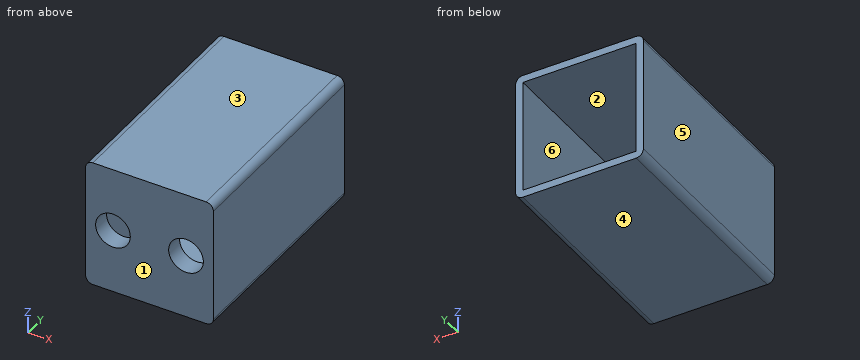
from build123d import *

# Parameters (mm, degrees)
SKETCH1_R           = 4.75
BOSS_EXTRUDE1_DEPTH = 60
SKETCH2_W           = 31
SKETCH2_H           = 31
CUT_EXTRUDE1_DEPTH  = 55


with BuildPart() as part:
    # Sketch1 → Boss-Extrude1 (new body)
    with BuildSketch(Plane(origin=(0, 0, 0), x_dir=(1, 0, 0), z_dir=(0, 1, 0))):
        with BuildLine():
            Line((2, 0), (33, 0))
            ThreePointArc((33, 0), (34.414213562, 0.585786438), (35, 2))
            Line((35, 2), (35, 33))
            ThreePointArc((35, 33), (34.414213562, 34.414213562), (33, 35))
            Line((33, 35), (2, 35))
            ThreePointArc((2, 35), (0.585786438, 34.414213562), (0, 33))
            Line((0, 33), (0, 2))
            ThreePointArc((0, 2), (0.585786438, 0.585786438), (2, 0))
        make_face()
        with Locations((7.5, 17.5)):
            Circle(SKETCH1_R, mode=Mode.SUBTRACT)
        with Locations((27.5, 17.5)):
            Circle(SKETCH1_R, mode=Mode.SUBTRACT)
    extrude(amount=BOSS_EXTRUDE1_DEPTH)

    # Sketch2 → Cut-Extrude1 (cut)
    with BuildSketch(Plane(origin=(0, 60, 0), x_dir=(1, 0, 0), z_dir=(0, 1, 0))):
        with Locations((17.5, 17.5)):
            Rectangle(SKETCH2_W, SKETCH2_H)
    extrude(amount=-CUT_EXTRUDE1_DEPTH, mode=Mode.SUBTRACT)


solid = part.part
CAD build for the part. Positions are in the model's coordinates, mm. Face numbers are marked on the shaded views. A direction names the side the tool comes from. Round coordinates to 2 decimals unless told otherwise and drop trailing zeros. Loops run counter-clockwise (first coordinate to the right, second up) from the corner with the lowest first, then second, coordinate; pieces in that order, holes last.
(1) Drop a flat-ended pin along its axis: pin 1 (1.5 mm diameter, centred on x = 29.5, z = -31.5, fed in from +Y). Give the stop position or say it passes through.
(2) Cut at D-D (z = -6.5). Give the cut face in (x, y), plus the area to 3 significant figures.
(3) Wall check: line 1 along X through (y, z) = (1.75, -17.5); line 2 along X through (y, z) = (9.5, -21.5); line 3 along Z through (x, y) = (7, 23). Give the ranges that are in metal, low to high.
(4) Which spindle directions (+Z, -Z, +X, -X, +Y, -Y) get a long thin tool onto all of the face, cutting with end or side? Do the marked faces 1 and 2. Say none if no direction does.
(5) Cut at A-A (x = 27.5). Give the cut face in (y, z), plus the area to 4 significant figures.
(6) Two-plate mould, pull along Z, no slides. Class the marked faces 3, 4, 5 and 6: +Z half, -Z half, draft (parallel to the pull), parting line (faces both ways), or undercut.
(7) Cut at C-C (y = 34.5). Give the cut face in (x, z), plus the area to 3 significant figures.
(8) Cut at B-B (z = -17.5). Give the cut face in (x, y).
Findings below:
1. pin 1: stops at y = 5
2. outline: (0, 0) - (35, 0) - (35, 60) - (33, 60) - (33, 5) - (2, 5) - (2, 60) - (0, 60) - close
2. area: 395 mm2
3. line 1: x = 0 to 2.75, 12.25 to 22.75, 32.25 to 35
3. line 2: x = 0 to 2, 33 to 35
3. line 3: z = -35 to -33, -2 to 0
4. face 1: +Z, -Z, +X, -X, -Y
4. face 2: +Y
5. outline: (0, -35) - (60, -35) - (60, -33) - (5, -33) - (5, -22.25) - (0, -22.25) - close; (0, -12.75) - (5, -12.75) - (5, -2) - (60, -2) - (60, 0) - (0, 0) - close
5. area: 347.5 mm2
6. face 3: +Z half
6. face 4: -Z half
6. face 5: draft
6. face 6: undercut
7. outline: (0, -33) arc R2 ccw to (2, -35) - (33, -35) arc R2 ccw to (35, -33) - (35, -2) arc R2 ccw to (33, 0) - (2, 0) arc R2 ccw to (0, -2) - close; hole (2, -33) - (33, -33) - (33, -2) - (2, -2) - close
7. area: 261 mm2
8. outline: (0, 0) - (2.75, 0) - (2.75, 5) - (2, 5) - (2, 60) - (0, 60) - close; (12.25, 0) - (22.75, 0) - (22.75, 5) - (12.25, 5) - close; (32.25, 0) - (35, 0) - (35, 60) - (33, 60) - (33, 5) - (32.25, 5) - close
